```python
from build123d import *

# Parameters (mm, degrees)
ESQUISSE1_W        = 190
ESQUISSE1_H        = 30
BOSS_EXTRU_1_DEPTH = 5
ESQUISSE2_R        = 1.5
ESQUISSE2_R_2      = 0.5
BOSS_EXTRU_2_DEPTH = 4
CONG_1_R           = 1


with BuildPart() as part:
    # Esquisse1 → Boss.-Extru.1 (new body)
    with BuildSketch(Plane.XY):
        Rectangle(ESQUISSE1_W, ESQUISSE1_H)
    extrude(amount=BOSS_EXTRU_1_DEPTH)

    # Esquisse2 → Boss.-Extru.2 (add)
    # profile 1 of 2: a face of its own
    with BuildSketch(Plane(origin=(0, 15, 0), x_dir=(1, 0, 0), z_dir=(0, 1, 0))):
        with Locations(Location((-52.5, -2.5, 0), (0, 0, 90))):
            Circle(ESQUISSE2_R)
        with Locations(Location((-52.5, -2.5, 0), (0, 0, 270))):
            Circle(ESQUISSE2_R_2, mode=Mode.SUBTRACT)
    # profile 2 of 2: a face of its own
    with BuildSketch(Plane(origin=(0, 15, 0), x_dir=(1, 0, 0), z_dir=(0, 1, 0))):
        with Locations(Location((52.5, -2.5, 0), (0, 0, 90))):
            Circle(ESQUISSE2_R)
        with Locations(Location((52.5, -2.5, 0), (0, 0, 90))):
            Circle(ESQUISSE2_R_2, mode=Mode.SUBTRACT)
    extrude(amount=BOSS_EXTRU_2_DEPTH)

    # Congé1
    cong_1_edges = [part.edges().sort_by_distance(p)[0] for p in [
        (-52.5, 19, 4),
        (52.5, 19, 4),
    ]]
    fillet(cong_1_edges, radius=CONG_1_R - 0.0001)  # a hair under: the kernel refuses the full size


solid = part.part
```
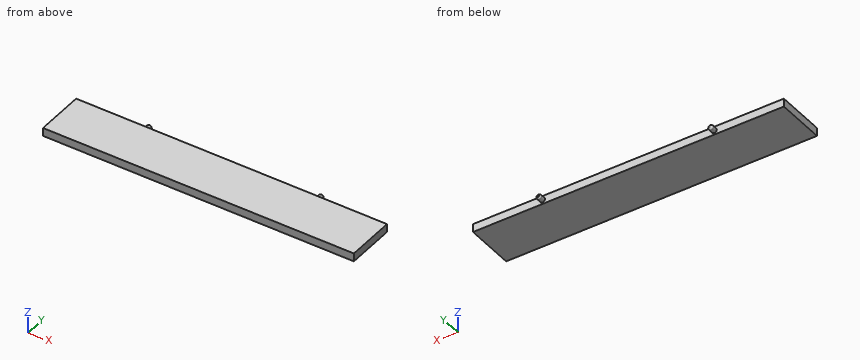
The model under review builds one solid part; all positions refer to its coordinate system, in mm. Round coordinates to 2 decimals unless told otherwise and drop trailing zeros. Write each loop counter-clockwise with the first axis right and the second up, starting at its lowest first coordinate (ties: lowest second). Pieces come first, ordered by that corner, then holes. Notation, with made-up numbers: M 31,73 L 71,73 A21 cw 71,77 Z; hole C 26,26.25 d11. An arc over 180 degrees is marked long. Use CSV: the item, a comma, the result in double quotes. Start each with the question number.
(1) Clearance check with a flat-ended pin moving along its axis: P1, Ø2, axis at x = -7, z = 2, coming from the +Y side. State where the tip first meets the part, or that it passes through.
(2) For line 1 along X through (y, z) = (17.15, 2.5); line 2 along Z through (x, y) = (52.5, 16.7); line 3 along Y through (x, z) = (11.5, 2.35), list the stretches that pass through material, from the lowest coordinate up.
(3) We need section A-A, the plane x = 29.5. State the section outline as (y, z) points.
Findings:
1,P1,"y = 15"
2,line 1,"-54 to -53, -52 to -51, 51 to 52, 53 to 54"
2,line 2,"1 to 2, 3 to 4"
2,line 3,"-15 to 15"
3,outline,"M -15,0 L 15,0 L 15,5 L -15,5 Z"
